```python
from build123d import *

# Parameters (mm, degrees)
BOSS_EXTRUDE1_DEPTH      = 3.5
BOSS_EXTRUDE1_DEPTH_BACK = 3.5
SKETCH1_R                = 1.6
CUT_EXTRUDE1_REACH       = 33.579
SKETCH3_R                = 1.6
SKETCH3_3_R              = 2.2
SKETCH3_3_R_2            = 1.6
CUT_EXTRUDE2_DEPTH       = 6
CUT_EXTRUDE3_REACH       = 33.579
FILLET1_R                = 2
FILLET2_R                = 0.4


with BuildPart() as part:
    # Sketch1 → Boss-Extrude1 (new, two sides: drawn at the far end of the back side and taken through both)
    with BuildSketch(Plane.XY.offset(-BOSS_EXTRUDE1_DEPTH_BACK)):
        with BuildLine():
            Line((-27, 8), (-18.64966284, 8))
            Line((-18.64966284, 8), (-10, -0.5))
            Line((-10, -0.5), (-3.979949748, -0.4))
            ThreePointArc((-3.979949748, -0.4), (0, -4), (3.979949748, -0.4))
            Line((3.979949748, -0.4), (6, -0.4))
            Line((6, -0.4), (6, 0.4))
            Line((6, 0.4), (3.979949748, 0.4))
            ThreePointArc((3.979949748, 0.4), (0, 4), (-3.979949748, 0.4))
            Line((-3.979949748, 0.4), (-10, 0.5))
            Line((-10, 0.5), (-16.848441102, 8))
            Line((-16.848441102, 8), (27, 8))
            Line((27, 8), (27, -8))
            Line((27, -8), (-27, -8))
            Line((-27, -8), (-27, 8))
        make_face()
        with Locations((-24, 0)):
            Circle(SKETCH1_R, mode=Mode.SUBTRACT)
        with Locations(Location((24, 0, 0), (0, 0, 180))):
            Circle(SKETCH1_R, mode=Mode.SUBTRACT)
    extrude(amount=BOSS_EXTRUDE1_DEPTH + BOSS_EXTRUDE1_DEPTH_BACK)

    # Cut-Extrude1: up to this plane
    cut_extrude1_end = Plane(origin=(-10, -0.5, -3.5), z_dir=(-0.016608865731892127, 0.9998620632762801, 0))
    # Sketch3 → Cut-Extrude1 (cut, up to the surface)
    with BuildSketch(Plane.XZ.offset(8), mode=Mode.PRIVATE) as cut_extrude1_sk1:
        with Locations(Location((-6.989974874, 0, 0), (0, 0, 270))):
            Circle(SKETCH3_R)
    cut_extrude1_tool1 = split(extrude(cut_extrude1_sk1.sketch, amount=-CUT_EXTRUDE1_REACH, mode=Mode.PRIVATE), bisect_by=cut_extrude1_end, keep=Keep.BOTH, mode=Mode.PRIVATE)
    add(cut_extrude1_tool1.solids().sort_by_distance((-6.989975, -8, 0))[0], mode=Mode.SUBTRACT)

    # Sketch3<3> → Cut-Extrude2 (cut)
    with BuildSketch(Plane.XZ.offset(8)):
        with Locations(Location((-6.989974874, 0, 0), (0, 0, 270))):
            Circle(SKETCH3_3_R)
        with Locations(Location((-6.989974874, 0, 0), (0, 0, 270))):
            Circle(SKETCH3_3_R_2, mode=Mode.SUBTRACT)
    extrude(amount=-CUT_EXTRUDE2_DEPTH, mode=Mode.SUBTRACT)

    # Cut-Extrude3: up to this plane
    cut_extrude3_end = Plane(origin=(-10, 0.5, -3.5), z_dir=(-0.016608865731892127, -0.9998620632762801, 0))
    # Sketch4 → Cut-Extrude3 (cut, up to the surface)
    with BuildSketch(Plane(origin=(0, 8, 0), x_dir=(1, 0, 0), z_dir=(0, 1, 0)), mode=Mode.PRIVATE) as cut_extrude3_sk1:
        with BuildLine():
            Line((-7.489974874, 1.6), (-6.489974874, 1.6))
            ThreePointArc((-6.489974874, 1.6), (-4.889974874, 0), (-6.489974874, -1.6))
            Line((-6.489974874, -1.6), (-7.489974874, -1.6))
            ThreePointArc((-7.489974874, -1.6), (-9.089974874, 0), (-7.489974874, 1.6))
        make_face()
    cut_extrude3_tool1 = split(extrude(cut_extrude3_sk1.sketch, amount=-CUT_EXTRUDE3_REACH, mode=Mode.PRIVATE), bisect_by=cut_extrude3_end, keep=Keep.BOTH, mode=Mode.PRIVATE)
    add(cut_extrude3_tool1.solids().sort_by_distance((-6.989975, 8, 0))[0], mode=Mode.SUBTRACT)

    # Fillet1
    fillet1_edges = [part.edges().sort_by_distance(p)[0] for p in [
        (27, 8, 0),
        (27, -8, 0),
        (-27, -8, 0),
        (-27, 8, 0),
    ]]
    fillet(fillet1_edges, radius=FILLET1_R)

    # Fillet2
    fillet2_edges = [part.edges().sort_by_distance(p)[0] for p in [
        (6, -0.4, 0),
        (6, 0.4, 0),
    ]]
    fillet(fillet2_edges, radius=FILLET2_R - 0.0001)  # a hair under: the kernel refuses the full size


solid = part.part
```
Design review of the part built by this model. Coordinates are the model's own, in mm. A direction names the side the tool comes from. Give positions to 0.01 mm unless a question says otherwise; leave off trailing zeros. Loops run counter-clockwise (first coordinate to the right, second up) from the corner with the lowest first, then second, coordinate; pieces in that order, holes last. Notation, with made-up numbers: M -31.5,36 L 14.5,36 A13 cw 14.5,54 Z; hole C 76,70 d6. An arc over 180 degrees is marked long. Return JSON: item names as keys, results as strings. Group by question number.
Item 1: Tool access review of faces 4 (the cylindrical face through (-9.138, -5.042, 0.477)), 5 (the cylindrical face through (0, 4, 0)), 6 (the flat face through (-7, 4, -1.6)), 7 (the cylindrical face through (-5.404, -1.22, 0.208)): name each direction out of +Z, -Z, +X, -X, +Y, -Y from which nothing blocks a thin tool from reaching the whole face with its end or side.
Item 2: Insertion check: pin 1 Ø4 at (x, z) = (-6.99, 0) entering from -Y. The pin has a flat end and moves straight along its axis. Give the tip position at first contact, or say it passes through.
Item 3: We need section A-A (x = -24). Give the boundary of the cut face in (y, z).
Item 4: For probe 1 along Y at (x, z) = (0.5, -1.5); probe 2 along Y at (x, z) = (24, 1); probe 3 along X at (y, z) = (4.5, 0.5), list the stretches that pass through material, from the lowest coordinate up.
Item 5: We need section B-B (z = 0.5). Give the number of separate pieces and of enclosed holes in the cut face, and give its area (3 significant figures).
Item 6: We need section C-C (y = 7.25). Give the boundary of the cut face in (x, z), and give its area (3 significant figures).
Item 7: Mouldability with a two-part tool opening along Y and no side actions: class faces 1 (the cylindrical face through (-26.4, 7.43, 0.05)), 2 (the flat face through (0, -8, 0)), 3 (the flat face through (5, -0.4, 0)) as released by +Y, released by -Y, zero draft, split by the parting line, or undercut.
Output:
{
 "1": {"face 4": "-Y", "face 5": "+Z, -Z", "face 6": "+Y", "face 7": "+Y, -Y"},
 "2": {"pin 1": "stops at y = -2"},
 "3": {"outline": "M -8,-3.5 L -1.6,-3.5 L -1.6,3.5 L -8,3.5 Z; M 1.6,-3.5 L 8,-3.5 L 8,3.5 L 1.6,3.5 Z"},
 "4": {"probe 1": "y = -8 to -3.97, 3.97 to 8", "probe 2": "y = -8 to -1.6, 1.6 to 8", "probe 3": "x = -27 to -15.09, -13.65 to -9.01, -4.97 to 27"},
 "5": {"separate pieces": "3", "enclosed holes": "2", "area": "715 mm^2"},
 "6": {"outline": "M -26.56,-3.5 L -17.89,-3.5 L -17.89,3.5 L -26.56,3.5 Z; M -16.16,-3.5 L 26.56,-3.5 L 26.56,3.5 L -16.16,3.5 Z; hole M -7.49,-1.6 L -6.49,-1.6 A1.6 ccw -6.49,1.6 L -7.49,1.6 A1.6 ccw Z", "area": "349 mm^2"},
 "7": {"face 1": "released by +Y", "face 2": "released by -Y", "face 3": "undercut"}
}
